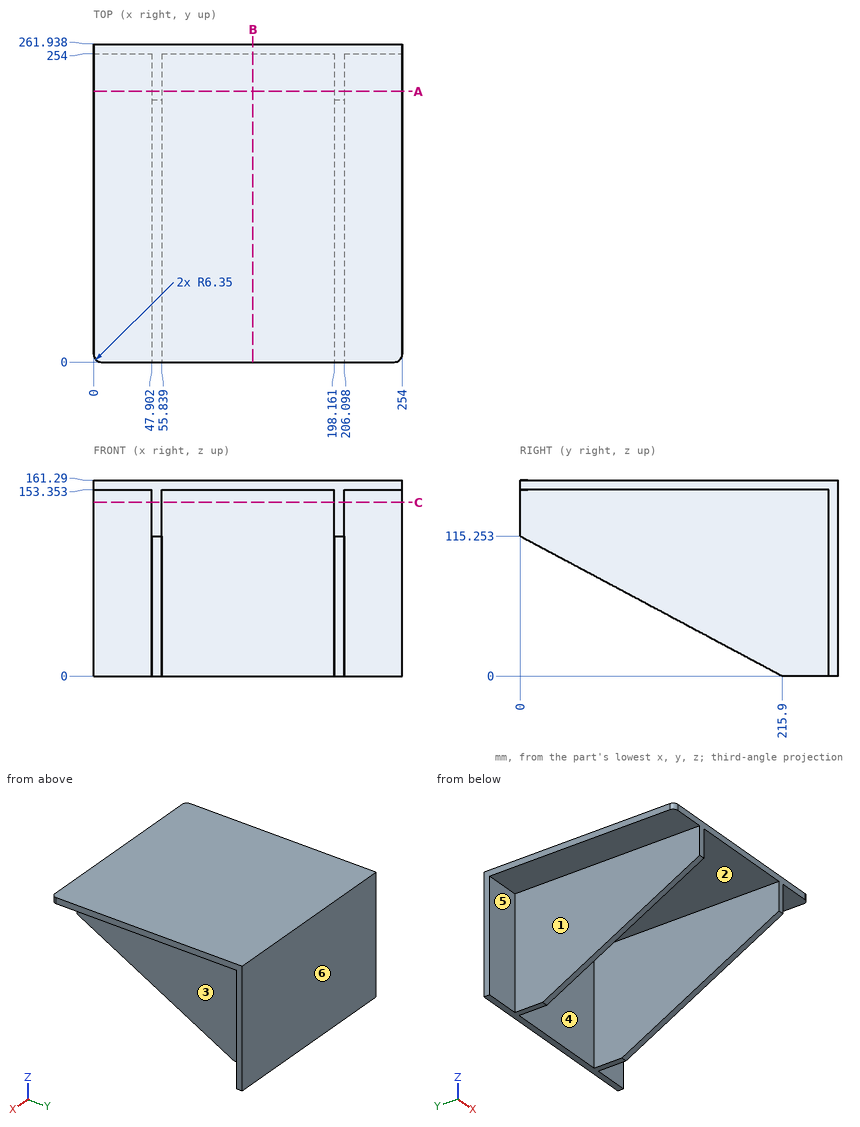
Geometry check sheet. Reference: drawing and pictorial views, mm from the part's lowest x, y, z. A direction names the side the tool comes from. Give positions to 0.01 mm unless a question says otherwise; leave off trailing zeros. Write each loop counter-clockwise with the first axis right and the second up, starting at its lowest first coordinate (ties: lowest second). Pieces come first, ordered by that corner, then holes. Notation, with made-up numbers: (4.5, -26.75) - (30.5, -26.75) arc R30 cw to (30.5, 10.25) - close; hole circle Ø5 at (-28, 22). An arc over 180 degrees is marked (long way). Put each result on its own line as item: value.
Q1. Section check C-C on z = 143. Record the cut outline in (x, y).
Result:
outline: (0, 254) - (47.9, 254) - (47.9, 0) - (55.84, 0) - (55.84, 254) - (198.16, 254) - (198.16, 0) - (206.1, 0) - (206.1, 254) - (254, 254) - (254, 261.94) - (0, 261.94) - close
Q2. Section check A-A on y = 223. Record the cut outline in (x, z), and give its area (3 significant figures).
Result:
outline: (0, 153.35) - (47.9, 153.35) - (47.9, 0) - (55.84, 0) - (55.84, 153.35) - (198.16, 153.35) - (198.16, 0) - (206.1, 0) - (206.1, 153.35) - (254, 153.35) - (254, 161.29) - (0, 161.29) - close
area: 4,450 mm2
Q3. Section check B-B on x = 131. Record the cut outline in (y, z), and give its area (3 significant figures).
Result:
outline: (0, 153.35) - (254, 153.35) - (254, 0) - (261.94, 0) - (261.94, 161.29) - (0, 161.29) - close
area: 3,300 mm2
Q4. Depth check by flat-ended pin: P1, Ø14.5, axis at x = 225, z = 52.5, coming from the -Y side; P2, Ø14.5, axis at x = 239.5, y = 117.5, coming from the -Z side; P3, Ø6, axis at y = 168.5, z = 66, coming from the -X side. Enter the tip coordinate at first touch or a pass-through.
Result:
P1: y = 254
P2: z = 153.35
P3: x = 47.9
Q5. Scan lines: probe 1 along X at (y, z) = (211.5, 80); probe 2 along Y at (x, z) = (74, 130); probe 3 along Z at (x, y) = (185.5, 177.5). Record each from-to range of solid material in increasing order. Write a range as from..to.
Result:
probe 1: 47.9..55.84, 198.16..206.1
probe 2: 254..261.94
probe 3: 153.35..161.29
Q6. Mould release check, pull along X, two halves, no side actions. Record for the marked faces 1, 2 and 3: released by +X, released by -X, zero draft, split by the parting line, or undercut.
Result:
face 1: released by -X
face 2: undercut
face 3: released by +X
Q7. Set-up check for the marked faces 4, 5 and 6: record each of +Z, -Z, +X, -X, +Y, -Y from which the full face is reachable in a straight line by a thin tool's end or side.
Result:
face 4: -Z, -Y
face 5: -Z, -X, -Y
face 6: +Z, -Z, +X, -X, +Y
